Part model, mm, in its own coordinate system. A direction names the side the tool comes from. Round coordinates to 2 decimals unless told otherwise and drop trailing zeros. Loops run counter-clockwise (first coordinate to the right, second up) from the corner with the lowest first, then second, coordinate; pieces in that order, holes last.
1) Mould opens along X. For faces 3 (the flat face through (2, 0, 1)), 4 (the cylindrical face through (-11.99, 0.53, 2.46)), 5 (the flat face through (3, 11, 5)) say: +X half, -X half, draft (parallel to the pull), parting line (faces both ways), or undercut.
2) Band-saw the part on A-A, the plane z = 2.45. Write the cut outline in (x, y), then the cut area to 3 significant figures.
3) 3-axis set-ups, long thin cutter, end or side, ignore diameter. For faces 1 (the flat face through (0, 0, 3)), 2 (the flat face through (0, 0, 0)): which of +Z, -Z, +X, -X, +Y, -Y reach the whole face in a straight line?
4) Probe line 1 (Y direction, x = 0, z = 2.1); line 2 (Y direction, x = 0, z = 3.05); line 3 (Z direction, x = 4.75, y = 1.5). List the from-to ranges inside material, lowest first.
5) Band-saw the part on D-D, the plane x = 5.5. Write the cut outline in (y, z), then the cut area to 3 significant figures.
6) Band-saw the part on B-B, the plane x = 0. Write the cut outline in (y, z), then the cut area to 3 significant figures.
7) Drop flat-ended pins along their axis: P1, Ø1.2, axis at x = 0, y = 0, coming from the +Z side; P2, Ø7, axis at x = -3.5, y = 5, coming from the +Z side; P3, Ø1, axis at y = 4.5, z = 0.5, coming from the -X side. Give the stop position or say it passes through.
from build123d import *

# Parameters (mm, degrees)
F0_R     = 11.75
F1_DEPTH = 1
F2_R     = 12
F2_R_2   = 11.25
F3_DEPTH = 5
F4_R     = 0.75
F5_DEPTH = 3


with BuildPart() as f1:
    # F0 (on Top) → F1 (new body)
    with BuildSketch(Plane.XY):
        Circle(F0_R)
    extrude(amount=F1_DEPTH)

    # F2 (on Top) → F3 (join)
    with BuildSketch(Plane.XY):
        Circle(F2_R)
        Circle(F2_R_2, mode=Mode.SUBTRACT)
    extrude(amount=F3_DEPTH)

    # F4 (on Top) → F5 (join)
    with BuildSketch(Plane.XY):
        Circle(F4_R)
    extrude(amount=F5_DEPTH)


solid = f1.part
Reported:
1. face 3: undercut
1. face 4: parting line
1. face 5: draft
2. outline: circle Ø24 at (0, 0); circle Ø1.5 at (0, 0); hole circle Ø22.5 at (0, 0)
2. area: 56.5 mm2
3. face 1: +Z
3. face 2: -Z, +X, -X, +Y, -Y
4. line 1: y = -12 to -11.25, -0.75 to 0.75, 11.25 to 12
4. line 2: y = -12 to -11.25, 11.25 to 12
4. line 3: z = 0 to 1
5. outline: (-10.67, 0) - (10.67, 0) - (10.67, 5) - (9.81, 5) - (9.81, 1) - (-9.81, 1) - (-9.81, 5) - (-10.67, 5) - close
5. area: 28.1 mm2
6. outline: (-12, 0) - (12, 0) - (12, 5) - (11.25, 5) - (11.25, 1) - (0.75, 1) - (0.75, 3) - (-0.75, 3) - (-0.75, 1) - (-11.25, 1) - (-11.25, 5) - (-12, 5) - close
6. area: 33.0 mm2
7. P1: stops at z = 3
7. P2: stops at z = 1
7. P3: stops at x = -11.31
